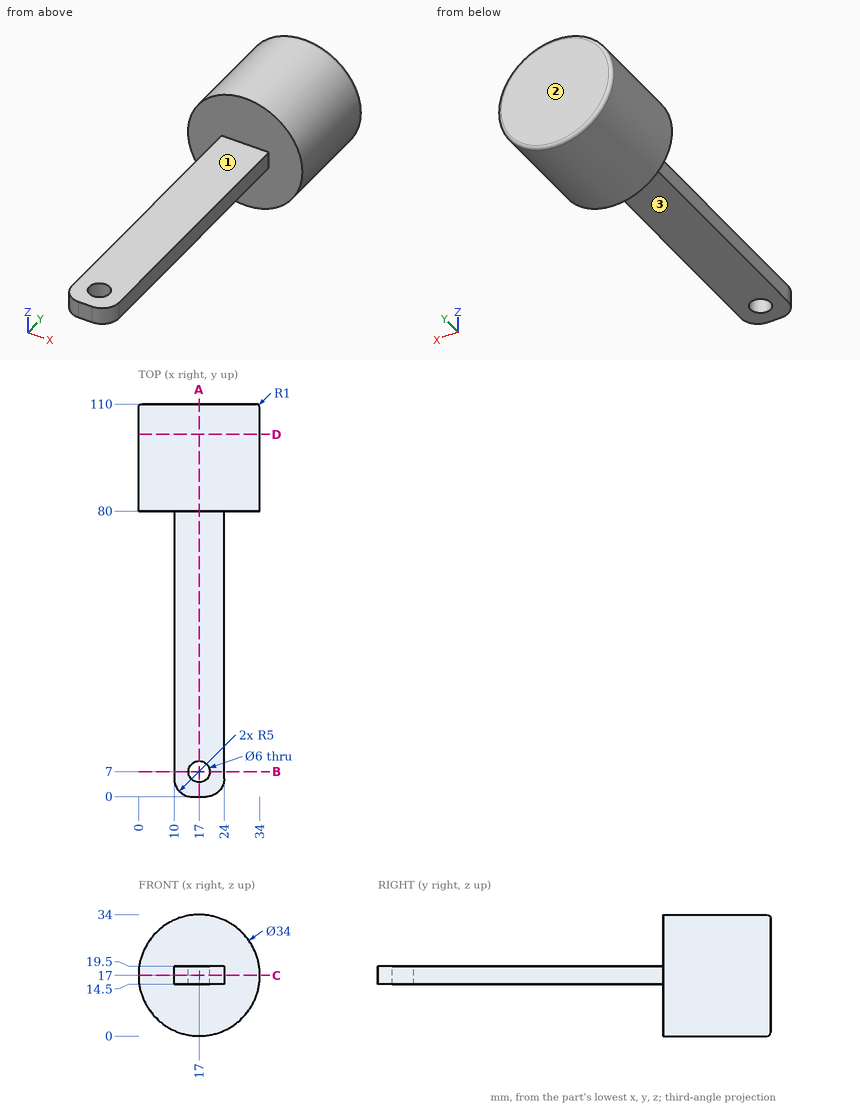
Verification items for this drawing (mm, ordinates from the low corner). A direction names the side the tool comes from. Round coordinates to 2 decimals unless told otherwise and drop trailing zeros. Order: outer loops, then holes, each group sorted by start corner. A loop starts at its lowest first (then second) coordinate and runs counter-clockwise, first axis right, second up. Notation, with made-up numbers: (-23.75, 54.5) -> (-0.75, 54.5) arc R20 ccw to (-0.75, 84.5) -> close; hole circle Ø8 at (-39, -15.75). An arc over 180 degrees is marked (long way). Use one line per item in the form item = value.
1. Cross-section at B-B, the plane y = 7. Enter the section's corners in (x, z).
Working result:
outline = (10, 14.5) -> (14, 14.5) -> (14, 19.5) -> (10, 19.5) -> close; (20, 14.5) -> (24, 14.5) -> (24, 19.5) -> (20, 19.5) -> close
2. Cross-section at A-A, the plane x = 17. Enter the section's corners in (y, z).
Working result:
outline = (0, 14.5) -> (4, 14.5) -> (4, 19.5) -> (0, 19.5) -> close; (10, 14.5) -> (80, 14.5) -> (80, 0) -> (109, 0) arc R1 ccw to (110, 1) -> (110, 33) arc R1 ccw to (109, 34) -> (80, 34) -> (80, 19.5) -> (10, 19.5) -> close
3. Cross-section at C-C, the plane z = 17. Enter the section's corners in (x, y), plus the area to 3 significant figures.
Working result:
outline = (0, 80) -> (10, 80) -> (10, 5) arc R5 ccw to (15, 0) -> (19, 0) arc R5 ccw to (24, 5) -> (24, 80) -> (34, 80) -> (34, 109) arc R1 ccw to (33, 110) -> (1, 110) arc R1 ccw to (0, 109) -> close; hole circle Ø6 at (17, 7)
area = 2,100 mm^2
4. Cross-section at D-D, the plane y = 101.5. Enter the section's corners in (x, z).
Working result:
outline = circle Ø34 at (17, 17)
5. Scan lines: line 1 along Y through (x, z) = (17, 17); line 2 along X through (y, z) = (7, 17); line 3 along Y through (x, z) = (26.5, 26.5). Record each from-to range of solid material in increasing order. Write a range as from..to.
Working result:
line_1 = 0..4, 10..110
line_2 = 10..14, 20..24
line_3 = 80..110
6. Set-up check for the marked faces 1, 2 and 3: record each of +Z, -Z, +X, -X, +Y, -Y from which the full face is reachable in a straight line by a thin tool's end or side.
Working result:
face_1 = +Z, +X, -X, -Y
face_2 = +Z, -Z, +X, -X, +Y
face_3 = -Z, +X, -X, -Y
7. Go/stop test with flat-tipped pins: pin 1 (5.5 mm diameter, centred on y = 58.5, z = 16, fed in from +X); pin 2 (15.5 mm diameter, centred on x = 13.5, y = 55, fed in from -Z); pin 3 (10 mm diameter, centred on x = 15, y = 15, fed in from +Z); pin 4 (3.5 mm diameter, centred on x = 17, y = 7, fed in from -Z). Record where each tip stops, or that it passes through.
Working result:
pin_1 = 24
pin_2 = 14.5
pin_3 = 19.5
pin_4 = through
